Geometry check sheet. Reference: the model listing, model coordinates, mm. Face numbers are marked on the shaded views. A direction names the side the tool comes from. Coordinates: 2 decimals unless noted, no trailing zeros. Write each loop counter-clockwise with the first axis right and the second up, starting at its lowest first coordinate (ties: lowest second). Pieces come first, ordered by that corner, then holes. Notation, with made-up numbers: (65.5, 72) -> (100.5, 72) arc R16 cw to (100.5, 76) -> close; hole circle Ø8 at (26, -38). An arc over 180 degrees is marked (long way). Answer as CSV lines item,"result".
Solid Edge part; units mm, degrees
sketch "Sketch1" plane through (0, 0, 0) normal (0, 0, 1) x (1, 0, 0)
  line L0 (-35, 6) -> (-2.3292, 6)
  line L1 (-2.3292, 6) -> (8.7613, 16.1389)
  line L2 (8.7613, 33.4946) -> (8.7613, 16.1389)
  line L3 (14.7613, 33.4946) -> (8.7613, 33.4946)
  line L4 (14.7613, 13.4946) -> (14.7613, 33.4946)
  line L5 (0, 0) -> (14.7613, 13.4946)
  line L6 (0, 0) -> (-35, 0)
  line L7 (-35, 0) -> (-35, 6)
extrude "Protrusion1" add sketch "Sketch1" along normal blind 12
fillet "Redondeo_1" radius 5 4 edges at (14.7613, 13.4946, 6) (0, 0, 6) (-2.3292, 6, 6) (8.7613, 16.1389, 6)
fillet "Redondeo_2" radius 6 4 edges at (11.7613, 33.4946, 12) (11.7613, 33.4946, 0) (-35, 3, 12) (-35, 3, 0)
sketch "Sketch2" plane through (-15.9705, 0, 6) normal (0, -1, 0) x (1, 0, 0)
  circle A0 centre (-13.0295, 0) radius 2.5
extrude "VaciadoExtruido_1" cut sketch "Sketch2" against normal blind 21.8267
sketch "Sketch3" plane through (14.7613, 24.5964, 6) normal (1, 0, 0) x (0, 1, 0)
  circle A0 centre (2.8982, 0) radius 2.5
extrude "VaciadoExtruido_2" cut sketch "Sketch3" against normal blind 18.7725
sketch "Sketch4" plane through (14.7613, 24.5964, 6) normal (1, 0, 0) x (0, 1, 0)
  circle A0 centre (2.8982, 0) radius 2.5
extrude "ProtrusiónExtruida_2" add sketch "Sketch4" along normal mid plane 12
sketch "Sketch5" plane through (14.7613, 24.5964, 6) normal (1, 0, 0) x (0, 1, 0)
  circle A0 centre (2.8982, 0) radius 2.5
extrude "VaciadoExtruido_3" cut sketch "Sketch5" along normal mid plane 37.0413
sketch "Sketch6" plane through (14.7613, 24.5964, 6) normal (1, 0, 0) x (0, 1, 0)
  circle A0 centre (2.8982, 0) radius 2.5
extrude "ProtrusiónExtruida_3" add sketch "Sketch6" along normal mid plane 12
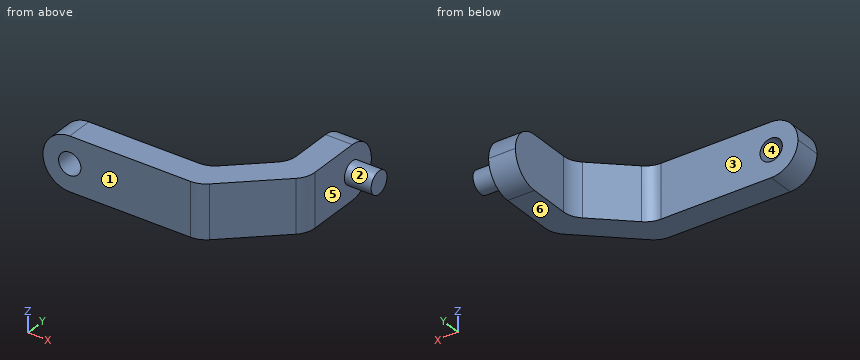
Item 1: Cross-section at C-C, the plane y = 21.5. Record the cut outline in (x, z).
Responses:
outline,"(8.76, 0) -> (14.76, 0) -> (14.76, 12) -> (8.76, 12) -> close"
Item 2: Thickness scan on probe 1 along Z at (x, y) = (-29, 4.65); probe 2 along X at (y, z) = (30, 3.25); probe 3 along Y at (x, z) = (-29, 11.75). Record the ranges inside material, lowest first.
Responses:
probe 1,"z = 0 to 3.5, 8.5 to 12"
probe 2,"x = 8.76 to 14.76"
probe 3,"y = 0 to 6"
Item 3: Cross-section at A-A, the plane x = -24. Record the cut outline in (y, z), plus the area to 3 significant figures.
Responses:
outline,"(0, 0) -> (6, 0) -> (6, 12) -> (0, 12) -> close"
area,"72.0 mm2"
Item 4: Release check for a two-part mould opening along X. For the marked faces 4, 5 and 6 record: +X half, -X half, draft (parallel to the pull), parting line (faces both ways), or undercut.
Responses:
face 4,"undercut"
face 5,"+X half"
face 6,"draft"
Item 5: Cross-section at D-D, the plane y = 26. Record the cut outline in (x, z), plus the area to 3 significant figures.
Responses:
outline,"(8.76, 0) -> (14.76, 0) -> (14.76, 4) -> (20.76, 4) -> (20.76, 8) -> (14.76, 8) -> (14.76, 12) -> (8.76, 12) -> close"
area,"96.0 mm2"
Item 6: Set-up check for the marked faces 1, 2 and 3: record each of +Z, -Z, +X, -X, +Y, -Y from which the full face is reachable in a straight line by a thin tool's end or side.
Responses:
face 1,"+Z, -Z, +X, -X, -Y"
face 2,"+X"
face 3,"+Z, -Z, -X, +Y"
Item 7: Depth check by flat-ended pin: pin 1 Ø3 at (y, z) = (20.5, 4.5) entering from -X; pin 2 Ø6 at (x, z) = (10, 3.5) entering from -Y. Enter the tip coordinate at first touch or a pass-through.
Responses:
pin 1,"stops at x = 8.76"
pin 2,"stops at y = 6.4"
Item 8: Cross-section at B-B, the plane z = 1.5. Record the cut outline in (x, y).
Responses:
outline,"(-32.97, 0) -> (-1.94, 0) arc R5 ccw to (1.43, 1.31) -> (13.13, 12.01) arc R5 ccw to (14.76, 15.7) -> (14.76, 31.46) -> (8.76, 31.46) -> (8.76, 18.34) arc R5 cw to (7.13, 14.65) -> (-0.9, 7.31) arc R5 cw to (-4.27, 6) -> (-32.97, 6) -> close"
